Autodesk Fusion 360 part; units mm, degrees
sketch "Sketch1" plane through (0, 0, 0) normal (0, 1, 0) x (1, 0, 0)
  line L0 (0, 0) -> (40, 0)
  line L1 (40, 0) -> (40, -10)
  line L2 (40, -10) -> (0, -10)
  line L3 (0, -10) -> (0, 0)
  dimension "d1" = 40
  dimension "d2" = 10
extrude "Extrude1" add sketch "Sketch1" along normal blind 6.35
sketch "Sketch2" plane through (0, 6.35, 0) normal (0, 1, 0) x (-1, 0, 0)
  line L0 (0, 10) -> (-40, 10)
  line L1 (-40, 10) -> (-40, 0)
  line L2 (-40, 0) -> (0, 0)
  line L3 (0, 0) -> (0, 10)
  line L4 (0, 5) -> (-40, 5) construction
  point P0 (-20, 5)
hole "Hole1" at (20, 6.35, 5) direction (0, -1, 0) diameter 3.3 end through all counterbore diameter 6.5 counterbore depth 3
sketch "Sketch3" plane through (0, 0, 10) normal (0, 0, 1) x (1, 0, 0)
  line L0 (0, 0) -> (40, 0)
  line L1 (40, 0) -> (40, 6.35)
  line L2 (40, 6.35) -> (0, 6.35)
  line L3 (0, 6.35) -> (0, 0)
  line L4 (0, 3.85) -> (39.5878, 3.85) construction
  point P0 (7.5, 3.85)
  point P1 (32.5, 3.85)
  dimension "d10" = 7.5
  dimension "d11" = 25
  dimension "d18" = 2.5
hole "Hole4" at (7.5, 3.85, 10) direction (0, 0, -1) diameter 2.5 end through all
hole "Hole5" at (32.5, 3.85, 10) direction (0, 0, -1) diameter 2.5 end through all
hole "Hole2" [suppressed]
hole "Hole3" [suppressed]
Model file for the job. Use its own axes, mm. A direction names the side the tool comes from. Coordinates: 2 decimals unless noted, no trailing zeros. Write each loop counter-clockwise with the first axis right and the second up, starting at its lowest first coordinate (ties: lowest second). Pieces come first, ordered by that corner, then holes. Notation, with made-up numbers: (-8, 6.5) - (38, 6.5) arc R38 cw to (38, 45.5) - close; hole circle Ø8 at (1, 36). An arc over 180 degrees is marked (long way). One line per question, with ' | ' between items. Start each with the question number.
Q1. Pull direction Z, two halves, no side cores. Call faces 3 (the face through (20, 3, 0)), 4 (the face through (21.4, 3.35, 6.4)), 5 (the face through (19.7, 6.35, 1.6)): pulls with the +Z half, pulls with the -Z half, needs draft (parallel to the pull), parting line crosses it, or undercut.
Q2. 3-axis set-ups, long thin cutter, end or side, ignore diameter. For faces 1 (the face through (17.26, 4.83, 6.75)), 2 (the face through (20, 3, 10)): which of +Z, -Z, +X, -X, +Y, -Y reach the whole face in a straight line?
Q3. Pin check, flat tips, straight feed: pin 1 (2.5 mm diameter, centred on x = 20, z = 5, fed in from -Y); pin 2 (6 mm diameter, centred on x = 20, z = 5, fed in from +Y). Stop position of each tip, or through.
Q4. Cut at A-A, the plane y = 3.85. List the corners of the cut face in (x, z), then the cut area to 3 significant figures.
Q5. Cut at C-C, the plane y = 5.5. List the corners of the cut face in (x, z), then the cut area to 3 significant figures.
Q6. Cut at D-D, the plane x = 7.5. List the corners of the cut face in (y, z).
Q7. Cut at B-B, the plane x = 20. List the corners of the cut face in (y, z).
Q8. Drill centre lines: line 1 (X direction, y = 1.05, z = 5); line 2 (Y direction, x = 7.5, z = 5); line 3 (X direction, y = 3.85, z = 2.75). Where is each one in solid material? Low to high. Write a range as [from, to].
Answer below:
1) face 3: pulls with the -Z half | face 4: undercut | face 5: needs draft
2) face 1: +Y | face 2: +Z, +X, -X, +Y, -Y
3) pin 1: through | pin 2: y = 3.35
4) outline: (0, 0) - (6.25, 0) - (6.25, 10) - (0, 10) - close; (8.75, 0) - (31.25, 0) - (31.25, 10) - (8.75, 10) - close; (33.75, 0) - (40, 0) - (40, 10) - (33.75, 10) - close; hole circle Ø6.5 at (20, 5) | area: 317 mm^2
5) outline: (0, 0) - (40, 0) - (40, 10) - (0, 10) - close; hole circle Ø6.5 at (20, 5) | area: 367 mm^2
6) outline: (0, 0) - (2.6, 0) - (2.6, 10) - (0, 10) - close; (5.1, 0) - (6.35, 0) - (6.35, 10) - (5.1, 10) - close
7) outline: (0, 0) - (6.35, 0) - (6.35, 1.75) - (3.35, 1.75) - (3.35, 3.35) - (0, 3.35) - close; (0, 6.65) - (3.35, 6.65) - (3.35, 8.25) - (6.35, 8.25) - (6.35, 10) - (0, 10) - close
8) line 1: [0, 18.35], [21.65, 40] | line 2: [0, 2.6], [5.1, 6.35] | line 3: [0, 6.25], [8.75, 17.65], [22.35, 31.25], [33.75, 40]
